Check sheet for the drawn part. Datum: minimum x, y, z corner. Units: mm. Coordinates: 2 decimals unless noted, no trailing zeros. Loops run counter-clockwise (first coordinate to the right, second up) from the corner with the lowest first, then second, coordinate; pieces in that order, holes last. Notation, with made-up numbers: (81.25, -20) -> (104.25, -20) arc R23 cw to (104.25, 5) -> close; hole circle Ø4 at (-1, 75.5). An arc over 180 degrees is marked (long way). Use CSV: the item, a comma, the result in double quotes. Start each with the question number.
1. Sectioned sample at B-B, the plane z = 12.5. Record the cut outline in (x, y), and give its area (3 significant figures).
2. Sectioned sample at A-A, the plane x = 15. Record the cut outline in (y, z).
3. Sectioned sample at C-C, the plane y = 426. Record the cut outline in (x, z).
4. Gauge pin test, flat end, axial feed: pin 1 (4 mm diameter, centred on y = 124, z = 51, fed in from -X). Record the tip position at first contact, or that the pin passes through.
5. Thickness scan on L1, parallel to Y at x = 45, z = 16; L2, parallel to Y at x = 12, z = 5. Record the ranges inside material, lowest first.
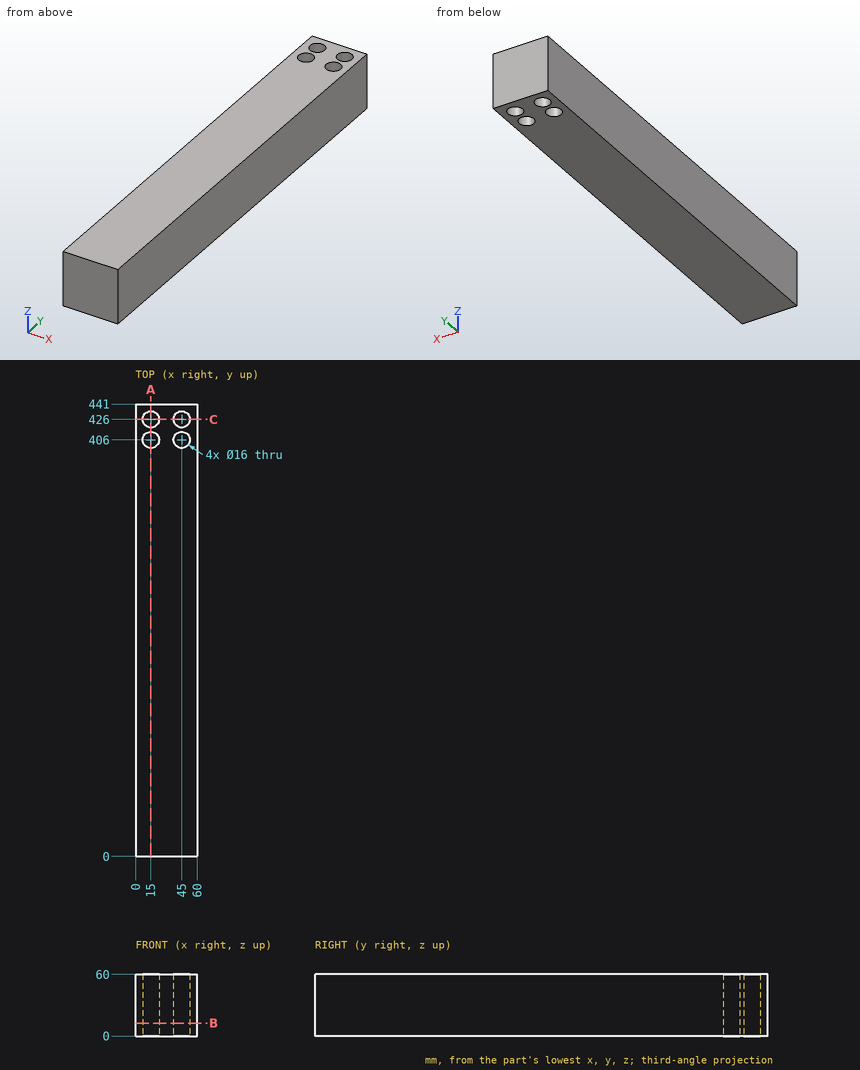
Completed:
1,outline,"(0, 0) -> (60, 0) -> (60, 441) -> (0, 441) -> close; hole circle Ø16 at (15, 406); hole circle Ø16 at (15, 426); hole circle Ø16 at (45, 406); hole circle Ø16 at (45, 426)"
1,area,"25,700 mm²"
2,outline,"(0, 0) -> (398, 0) -> (398, 60) -> (0, 60) -> close; (414, 0) -> (418, 0) -> (418, 60) -> (414, 60) -> close; (434, 0) -> (441, 0) -> (441, 60) -> (434, 60) -> close"
3,outline,"(0, 0) -> (7, 0) -> (7, 60) -> (0, 60) -> close; (23, 0) -> (37, 0) -> (37, 60) -> (23, 60) -> close; (53, 0) -> (60, 0) -> (60, 60) -> (53, 60) -> close"
4,pin 1,"x = 0"
5,L1,"0 to 398, 414 to 418, 434 to 441"
5,L2,"0 to 398.58, 413.42 to 418.58, 433.42 to 441"
